Source: CAD feature listing. Evaluate the final solid. Frame: model axes, mm. Face numbers are marked on the shaded views. A direction names the side the tool comes from. Give positions to 0.01 mm unless a question says otherwise; leave off trailing zeros. Loops run counter-clockwise (first coordinate to the right, second up) from the corner with the lowest first, then second, coordinate; pieces in that order, holes last. Notation, with made-up numbers: M -13,14 L 1,14 A24 ccw 1,39 Z; hole C 42,22.25 d10. An arc over 180 degrees is marked long. Answer in a Markdown table with one row per item.
```python
from build123d import *

# Parameters (mm, degrees)
ESQUISSE1_R             = 45
BOSS_EXTRU_1_DEPTH      = 50
ESQUISSE2_W             = 55.8
ESQUISSE2_H             = 56
ENL_V_MAT_EXTRU_1_DEPTH = 23
CONG_1_R                = 3
ESQUISSE3_W             = 12
ESQUISSE3_H             = 15
ENL_V_MAT_EXTRU_2_DEPTH = 81.932070281
CONG_2_R                = 3
CONG_3_R                = 3
CHANFREIN1_SIZE         = 1
ESQUISSE5_R             = 1.6
ENL_V_MAT_EXTRU_3_DEPTH = 81.932070281
ESQUISSE6_R             = 3.425
ESQUISSE6_R_2           = 1.6
ENL_V_MAT_EXTRU_4_DEPTH = 5
ESQUISSE7_R             = 2.6
ESQUISSE7_R_2           = 1.6
ENL_V_MAT_EXTRU_5_DEPTH = 30
CHANFREIN2_SIZE         = 1
ENL_V_START             = -4
ESQUISSE8_R             = 1.925
ESQUISSE8_R_2           = 1.6
ENL_V_MAT_EXTRU_6_DEPTH = 4


with BuildPart() as part:
    # Esquisse1 → Boss.-Extru.1 (new body)
    with BuildSketch(Plane.XY):
        Circle(ESQUISSE1_R)
    extrude(amount=BOSS_EXTRU_1_DEPTH)

    # Esquisse2 → Enlèv. mat.-Extru.1 (cut)
    with BuildSketch(Plane.XY.offset(50)):
        Rectangle(ESQUISSE2_W, ESQUISSE2_H)
    extrude(amount=-ENL_V_MAT_EXTRU_1_DEPTH, mode=Mode.SUBTRACT)

    # Congé1
    cong_1_edges = [part.edges().sort_by_distance(p)[0] for p in [
        (-27.9, -28, 38.5),
        (-27.9, 28, 38.5),
        (27.9, 28, 38.5),
        (27.9, -28, 38.5),
    ]]
    fillet(cong_1_edges, radius=CONG_1_R)

    # Esquisse3 → Enlèv. mat.-Extru.2 (cut, through all)
    with BuildSketch(Plane.XY.offset(50)):
        with Locations((0, -35.5)):
            Rectangle(ESQUISSE3_W, ESQUISSE3_H)
    extrude(amount=-ENL_V_MAT_EXTRU_2_DEPTH, mode=Mode.SUBTRACT)

    # Congé2
    cong_2_edges = [part.edges().sort_by_distance(p)[0] for p in [
        (-6, -28, 38.5),
        (6, -28, 38.5),
        (6, -43, 25),
        (-6, -43, 25),
    ]]
    fillet(cong_2_edges, radius=CONG_2_R)

    # Congé3
    cong_3_edges = [part.edges().sort_by_distance(p)[0] for p in [
        (6, -28, 13.5),
        (-6, -28, 13.5),
    ]]
    fillet(cong_3_edges, radius=CONG_3_R)

    # Chanfrein1
    chanfrein1_edges = [part.edges().sort_by_distance(p)[0] for p in [
        (27.9, 0, 50),
        (-16.95, -28, 50),
        (-27.9, 0, 50),
        (0, 28, 50),
        (27.021320344, -27.121320344, 50),
        (-27.021320344, -27.121320344, 50),
        (-27.021320344, 27.121320344, 50),
        (27.021320344, 27.121320344, 50),
        (16.95, -28, 50),
        (6, -35.5, 50),
        (0, -43, 50),
        (-6, -35.5, 50),
        (-6.878679656, -28.878679656, 50),
        (6.878679656, -28.878679656, 50),
        (5.121320344, -42.121320344, 50),
        (-5.121320344, -42.121320344, 50),
    ]]
    chamfer(chanfrein1_edges, length=CHANFREIN1_SIZE)

    # Esquisse5 → Enlèv. mat.-Extru.3 (cut, through all)
    with BuildSketch(Plane.XY.offset(50)):
        with Locations((-34.641016151, -20)):
            Circle(ESQUISSE5_R)
        with Locations((0, 40)):
            Circle(ESQUISSE5_R)
        with Locations((34.641016151, -20)):
            Circle(ESQUISSE5_R)
    extrude(amount=-ENL_V_MAT_EXTRU_3_DEPTH, mode=Mode.SUBTRACT)

    # Esquisse6 → Enlèv. mat.-Extru.4 (cut)
    # profile 1 of 3: a face of its own
    with BuildSketch(Plane.XY.offset(50)):
        with Locations((-34.641016151, -20)):
            Circle(ESQUISSE6_R)
        with Locations((-34.641016151, -20)):
            Circle(ESQUISSE6_R_2, mode=Mode.SUBTRACT)
    # profile 2 of 3: a face of its own
    with BuildSketch(Plane.XY.offset(50)):
        with Locations((0, 40)):
            Circle(ESQUISSE6_R)
        with Locations((0, 40)):
            Circle(ESQUISSE6_R_2, mode=Mode.SUBTRACT)
    # profile 3 of 3: a face of its own
    with BuildSketch(Plane.XY.offset(50)):
        with Locations((34.641016151, -20)):
            Circle(ESQUISSE6_R)
        with Locations((34.641016151, -20)):
            Circle(ESQUISSE6_R_2, mode=Mode.SUBTRACT)
    extrude(amount=-ENL_V_MAT_EXTRU_4_DEPTH, mode=Mode.SUBTRACT)

    # Esquisse7 → Enlèv. mat.-Extru.5 (cut)
    # profile 1 of 3: a face of its own
    with BuildSketch(Plane.XY.offset(50)):
        with Locations((-34.641016151, -20)):
            Circle(ESQUISSE7_R)
        with Locations((-34.641016151, -20)):
            Circle(ESQUISSE7_R_2, mode=Mode.SUBTRACT)
    # profile 2 of 3: a face of its own
    with BuildSketch(Plane.XY.offset(50)):
        with Locations((0, 40)):
            Circle(ESQUISSE7_R)
        with Locations((0, 40)):
            Circle(ESQUISSE7_R_2, mode=Mode.SUBTRACT)
    # profile 3 of 3: a face of its own
    with BuildSketch(Plane.XY.offset(50)):
        with Locations((34.641016151, -20)):
            Circle(ESQUISSE7_R)
        with Locations((34.641016151, -20)):
            Circle(ESQUISSE7_R_2, mode=Mode.SUBTRACT)
    extrude(amount=-ENL_V_MAT_EXTRU_5_DEPTH, mode=Mode.SUBTRACT)

    # Chanfrein2
    chanfrein2_edges = [part.edges().sort_by_distance(p)[0] for p in [
        (-36.241016151, -20, 20),
        (-1.6, 40, 20),
        (33.041016151, -20, 20),
    ]]
    chamfer(chanfrein2_edges, length=CHANFREIN2_SIZE - 0.0001)  # a hair under: the kernel refuses the full size

    # Esquisse8 → Enlèv. mat.-Extru.6 (cut)
    # profile 1 of 3: a face of its own
    with BuildSketch(Plane(origin=(0, 0, 0), x_dir=(-1, 0, 0), z_dir=(0, 0, -1)).offset(ENL_V_START)):
        with Locations((-34.641016151, -20)):
            Circle(ESQUISSE8_R)
        with Locations(Location((-34.641016151, -20, 0), (0, 0, 180))):
            Circle(ESQUISSE8_R_2, mode=Mode.SUBTRACT)
    # profile 2 of 3: a face of its own
    with BuildSketch(Plane(origin=(0, 0, 0), x_dir=(-1, 0, 0), z_dir=(0, 0, -1)).offset(ENL_V_START)):
        with Locations((0, 40)):
            Circle(ESQUISSE8_R)
        with Locations(Location((0, 40, 0), (0, 0, 180))):
            Circle(ESQUISSE8_R_2, mode=Mode.SUBTRACT)
    # profile 3 of 3: a face of its own
    with BuildSketch(Plane(origin=(0, 0, 0), x_dir=(-1, 0, 0), z_dir=(0, 0, -1)).offset(ENL_V_START)):
        with Locations((34.641016151, -20)):
            Circle(ESQUISSE8_R)
        with Locations(Location((34.641016151, -20, 0), (0, 0, 180))):
            Circle(ESQUISSE8_R_2, mode=Mode.SUBTRACT)
    extrude(amount=ENL_V_MAT_EXTRU_6_DEPTH, mode=Mode.SUBTRACT)


solid = part.part
```
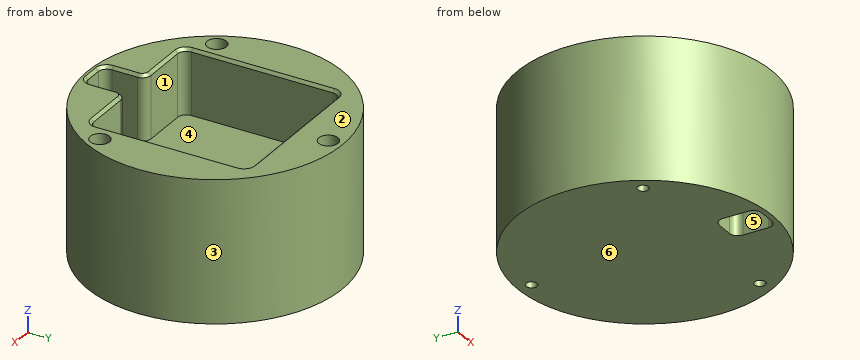
Q1. Mould query, pull axis Y, two halves, no side actions, for the marked faces 1, 2 and 3. Classes: +Y half, -Y half, draft (parallel to the pull), parting line (faces both ways), or undercut.
Values follow:
| item | result |
|---|---|
| face 1 | undercut |
| face 2 | draft |
| face 3 | parting line |
Q2. Contact query for flat-ended pins moving along their axis: pin 1 Ø6 at (x, y) = (0, 40) entering from -Z; pin 2 Ø4 at (x, y) = (-34.5, -20.5) entering from +Z; pin 3 Ø4.5 at (y, z) = (-34, 25.5) entering from +X; pin 4 Ø11 at (x, z) = (-0.5, 37) entering from -Y. Output: stop coordinate, or through.
Values follow:
| item | result |
|---|---|
| pin 1 | z = 0 |
| pin 2 | z = 19.92 |
| pin 3 | x = 31.89 |
| pin 4 | y = -45 |
Q3. Section query C-C (y = 0). Output: boundary loops of the cut face in (x, z), plus the area to 3 significant figures.
Values follow:
| item | result |
|---|---|
| outline | M -45,0 L 45,0 L 45,50 L 28.9,50 L 27.9,49 L 27.9,27 L -27.9,27 L -27.9,49 L -28.9,50 L -45,50 Z |
| area | 3,220 mm^2 |
Q4. Ray query, probe 1 along Y at (x, z) = (0, 40); probe 2 along Y at (x, z) = (0, 1) (3 decimals); probe 3 along X at (y, z) = (-19.5, 18). Return the intervals inside material, ascending. Write a range as from..to.
Values follow:
| item | result |
|---|---|
| probe 1 | -45..-43, 28..37.4, 42.6..45 |
| probe 2 | -45..-43, -28..38.075, 41.925..45 |
| probe 3 | -40.56..-36.16, -33.12..33.12, 36.16..40.56 |
Q5. Section query B-B (z = 22). Output: boundary loops of the cut face in (x, y).
Values follow:
| item | result |
|---|---|
| outline | C 0,0 d90; hole C -34.64,-20 d5.2; hole M -6,-40 A3 ccw -3,-43 L 3,-43 A3 ccw 6,-40 L 6,-31 A3 ccw 3,-28 L -3,-28 A3 ccw -6,-31 Z; hole C 0,40 d5.2; hole C 34.64,-20 d5.2 |
Q6. Reachability of the marked faces 4, 5 and 6 from +Z, -Z, +X, -X, +Y, -Y: full face, straight path, thin tool, end or side. Return the list, or none.
Values follow:
| item | result |
|---|---|
| face 4 | +Z |
| face 5 | +Z, -Z |
| face 6 | -Z, +X, -X, +Y, -Y |
Q7. Section query A-A (x = 0). Give the number of separate pieces and of enclosed holes in the cut face, plus the area to 3 significant figures.
Values follow:
| item | result |
|---|---|
| separate pieces | 3 |
| enclosed holes | 0 |
| area | 2,230 mm^2 |
